Could you check a few things on this model? Use its own coordinates, in mm. Face numbers are marked on the shaded views. A direction names the side the tool comes from. Coordinates: 2 decimals unless noted, no trailing zeros. Loops run counter-clockwise (first coordinate to the right, second up) from the corner with the lowest first, then second, coordinate; pieces in that order, holes last. Notation, with made-up numbers: (20.25, 13.25) - (25.25, 13.25) arc R21 ccw to (25.25, 25.25) - close; hole circle Ø8 at (0, 3.5). An arc over 180 degrees is marked (long way). One line per item, written item: value. Start each with the question number.
(1) If we section it at C-C on y = 12: Write out the boundary of the cut face in (x, z).
(2) I'm going to push flat-ended pins straight in: P1, Ø10, axis at y = 67, z = 12, coming from the -X side; P2, Ø25, axis at y = 81, z = 12, coming from the +X side; P3, Ø22.5, axis at x = 28.5, z = 11.5, coming from the +Y side. Where does each tip first touch, or does it pass through?
(3) If I drill on line 1 along Y through (x, z) = (10, 10); line 2 along Y through (x, z) = (8.5, 6.5); line 3 along Z through (x, y) = (3, 70), over which ranges is the centre line in solid material (lowest first)? Write a range as from..to.
(4) If we section it at A-A on x = 21: Write out the boundary of the cut face in (y, z).
(5) On a 3-axis mill with a long thin cutter (end or side, diameter ignored), from which of +Z, -Z, +X, -X, +Y, -Y can I reach the whole of each face in a straight line? I mean the marked faces 1, 2 and 3. Say none if no direction works.
(6) If we section it at B-B on z = -10: Write out the boundary of the cut face in (x, y), then the cut area to 3 significant figures.
(7) If we section it at D-D on z = 0: Write out the boundary of the cut face in (x, y), then the cut area to 3 significant figures.
(8) If we mould it in two halves opening along Z, with no side actions, what happens to the marked faces 4, 5 and 6? For each: pulls with the +Z half, pulls with the -Z half, needs draft (parallel to the pull), parting line crosses it, or undercut.
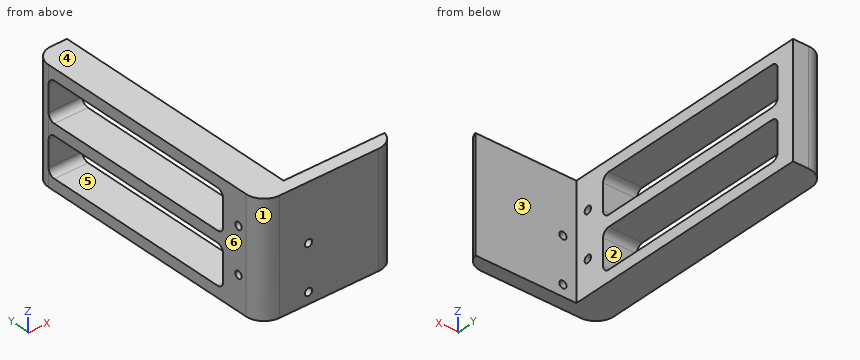
```python
from build123d import *

# Parameters (mm, degrees)
EXTRUDE_1_DEPTH     = 25
FILLET_1_R          = 8
SKETCH_2_R          = 1.65
CUT_EXTRUDE_1_DEPTH = 137.034003102
SKETCH_3_R          = 1.6
CUT_EXTRUDE_2_DEPTH = 131.794686436
SKETCH_4_W          = 17.5
SKETCH_4_H          = 91.5
CUT_EXTRUDE_3_DEPTH = 137.034003102
FILLET_2_R          = 3


with BuildPart() as part:
    # 草图1 → 凸台-拉伸1 (new, symmetric)
    with BuildSketch(Plane.XY):
        Polygon((0, 0), (0, 119.5), (15, 119.5), (15, 6), (60, 6), (60, 0), align=None)
    extrude(amount=EXTRUDE_1_DEPTH, both=True)

    # 圆角1
    # the kernel refuses this fillet: 8 mm, written as the material it takes off along each edge
    with BuildSketch(Plane(origin=(0, 119.5, 45), x_dir=(0, -1, 0), z_dir=(0, 0, -1)), Plane(origin=(0, 0, -45), x_dir=(0, 1, 0), z_dir=(0, 0, 1))) as fillet_1_piece_1:
        with BuildLine():
            CenterArc((FILLET_1_R, -FILLET_1_R), FILLET_1_R, 90, 90)
            Line((0, -FILLET_1_R), (-FILLET_1_R * 0.02, -FILLET_1_R))
            Line((-FILLET_1_R * 0.02, -FILLET_1_R), (-FILLET_1_R * 0.02, FILLET_1_R * 0.02))
            Line((-FILLET_1_R * 0.02, FILLET_1_R * 0.02), (FILLET_1_R, FILLET_1_R * 0.02))
            Line((FILLET_1_R, FILLET_1_R * 0.02), (FILLET_1_R, 0))
        make_face()
    extrude(amount=90, mode=Mode.SUBTRACT)
    with BuildSketch(Plane(origin=(60, 0, -44.364916731), x_dir=(0, 1, 0), z_dir=(0, 0, 1))) as fillet_1_piece_2:
        with BuildLine():
            CenterArc((8, 7.745966692), FILLET_1_R, 180, 75.522487814)
            Line((0, 7.745966692), (-0.16, 7.745966692))
            Line((-0.16, 7.745966692), (-0.16, 0))
            Line((-0.16, 0), (0, -0.16))
            ThreePointArc((0, -0.16), (3, -0.16), (5.96, -0.154919334))
            Line((5.96, -0.154919334), (6, 0))
        make_face()
    extrude(amount=88.729833462, mode=Mode.SUBTRACT)

    # 草图2 → 切除-拉伸1 (cut, through all)
    with BuildSketch(Plane.ZY):
        with Locations((10, 12)):
            Circle(SKETCH_2_R)
        with Locations((-10, 12)):
            Circle(SKETCH_2_R)
    extrude(amount=-CUT_EXTRUDE_1_DEPTH, mode=Mode.SUBTRACT)

    # 草图3 → 切除-拉伸2 (cut, through all)
    with BuildSketch(Plane(origin=(0, 6, 0), x_dir=(1, 0, 0), z_dir=(0, 1, 0))):
        with Locations(Location((21, 0, 0), (0, 0, 270))):
            Circle(SKETCH_3_R)
        with Locations(Location((21, 20, 0), (0, 0, 270))):
            Circle(SKETCH_3_R)
    extrude(amount=-CUT_EXTRUDE_2_DEPTH, mode=Mode.SUBTRACT)

    # 草图4 → 切除-拉伸3 (cut, through all)
    with BuildSketch(Plane.ZY):
        with Locations((-11.25, 65.75)):
            Rectangle(SKETCH_4_W, SKETCH_4_H)
        with Locations((11.25, 65.75)):
            Rectangle(SKETCH_4_W, SKETCH_4_H)
    extrude(amount=-CUT_EXTRUDE_3_DEPTH, mode=Mode.SUBTRACT)

    # 圆角2
    fillet_2_edges = [part.edges().sort_by_distance(p)[0] for p in [
        (7.5, 111.5, -20),
        (7.5, 20, -2.5),
        (7.5, 20, -20),
        (7.5, 111.5, -2.5),
        (7.5, 111.5, 2.5),
        (7.5, 20, 20),
        (7.5, 20, 2.5),
        (7.5, 111.5, 20),
    ]]
    fillet(fillet_2_edges, radius=FILLET_2_R)


solid = part.part
```
Values:
1. outline: (0, -25) - (15, -25) - (15, -11.65) - (0, -11.65) - close; (0, -8.35) - (15, -8.35) - (15, 8.35) - (0, 8.35) - close; (0, 11.65) - (15, 11.65) - (15, 25) - (0, 25) - close
2. P1: passes through
2. P2: stops at x = 15
2. P3: stops at y = 6
3. line 1: y = 0..10.35, 13.65..20, 111.5..119.5
3. line 2: y = 0..20, 111.5..119.5
3. line 3: z = -25..-20, -2.5..2.5, 20..25
4. outline: (0, -25) - (6, -25) - (6, -21.6) - (0, -21.6) - close; (0, -18.4) - (6, -18.4) - (6, -1.6) - (0, -1.6) - close; (0, 1.6) - (6, 1.6) - (6, 25) - (0, 25) - close
5. face 1: +Z, -Z, -X, -Y
5. face 2: +X, -X
5. face 3: +Z, -Z, +X, +Y
6. outline: (0, 8) arc R8 ccw to (8, 0) - (52.25, 0) arc R8 ccw to (60, 6) - (15, 6) - (15, 10.35) - (0, 10.35) - close; (0, 13.65) - (15, 13.65) - (15, 20) - (0, 20) - close; (0, 111.5) - (15, 111.5) - (15, 119.5) - (8, 119.5) arc R8 ccw to start
6. area: 601 mm2
7. outline: (0, 8) arc R8 ccw to (8, 0) - (19.4, 0) - (19.4, 6) - (15, 6) - (15, 119.5) - (8, 119.5) arc R8 ccw to (0, 111.5) - close; (22.6, 0) - (52.25, 0) arc R8 ccw to (60, 6) - (22.6, 6) - close
7. area: 2,000 mm2
8. face 4: pulls with the +Z half
8. face 5: undercut
8. face 6: needs draft
